Here's how the part is built. I have some questions about the finished solid (model axes, mm). A direction names the side the tool comes from. Round coordinates to 2 decimals unless told otherwise and drop trailing zeros. Loops run counter-clockwise (first coordinate to the right, second up) from the corner with the lowest first, then second, coordinate; pieces in that order, holes last. Notation, with made-up numbers: (-40, 37) -> (-1, 37) arc R12 cw to (-1, 51) -> close; hole circle Ø11 at (-4.75, -33.75). An arc over 180 degrees is marked (long way). Use one line per item in the form item = value. Start each with the question number.
Item 1: If we section it at A-A (z = 8.25): Write out the boundary of the cut face in (x, y), then the cut area to 3 significant figures.
Item 2: If we section it at B-B (x = -3.75): Write out the boundary of the cut face in (y, z), then the cut area to 3 significant figures.
Item 3: If we section it at D-D (x = 11): Write out the boundary of the cut face in (y, z).
Item 4: If I drill on L1, parallel to Z at x = 10.75, y = -0.25; L2, parallel to Z at x = 8, y = -5.75; L3, parallel to X at y = -3.5, z = 4, over which ranges is the centre line in solid material (lowest first)? Write a range as [from, to].
Item 5: For faces 1 (the face through (-7.88, -7.32, 14.38)), 2 (the face through (-1.63, -7.32, 4.87)), 3 (the face through (-7.493, 0.33, 21.869)), 4 (the face through (9.119, 0.33, 20.243)), which set-ups out of +Z, -Z, +X, -X, +Y, -Y let a thin tool reach every point of the face, with its end or its side?
Item 6: I'm going to push flat-ended pins straight in: pin 1 Ø2 at (x, z) = (-1.5, 10) entering from -Y; pin 2 Ø4 at (x, y) = (7, -5.5) entering from +Z; pin 3 Ø1 at (x, z) = (4, 12) entering from +Y; pin 4 Ø1.5 at (x, z) = (2, 22.5) entering from +Y. Where does each tip first touch, or does it pass through?
Item 7: If we section it at C-C (y = 0): Write out the boundary of the cut face in (x, z).
```python
from build123d import *

# Parameters (mm, degrees)
SKETCH1_R                = 7.5
BOSS_EXTRUDE1_DEPTH      = 25.5
BOSS_EXTRUDE2_DEPTH      = 12.75
BOSS_EXTRUDE2_DEPTH_BACK = 12.75
SKETCH2_R                = 7.5


with BuildPart() as part:
    # Sketch1 → Boss-Extrude1 (new body)
    with BuildSketch(Plane.XY):
        Circle(SKETCH1_R)
    extrude(amount=BOSS_EXTRUDE1_DEPTH)

    # Sketch2 → Boss-Extrude2 (add, two sides: drawn at the far end of the back side and taken through both)
    with BuildSketch(Plane(origin=(0, 0, 0), x_dir=(0, 0, -1), z_dir=(1, 0, 0)).offset(-BOSS_EXTRUDE2_DEPTH_BACK)):
        with Locations((-12.75, 0)):
            Circle(SKETCH2_R)
    extrude(amount=BOSS_EXTRUDE2_DEPTH + BOSS_EXTRUDE2_DEPTH_BACK)


solid = part.part
```
Values found:
q1.outline = (-12.75, -6) -> (-4.5, -6) arc R7.5 ccw to (4.5, -6) -> (12.75, -6) -> (12.75, 6) -> (4.5, 6) arc R7.5 ccw to (-4.5, 6) -> (-12.75, 6) -> close
q1.area = 324 mm2
q2.outline = (-6.5, 0) -> (6.5, 0) -> (6.5, 9) arc R7.5 ccw to (6.5, 16.5) -> (6.5, 25.5) -> (-6.5, 25.5) -> (-6.5, 16.5) arc R7.5 ccw to (-6.5, 9) -> close
q2.area = 341 mm2
q3.outline = circle Ø15 at (0, 12.75)
q4.L1 = [5.25, 20.25]
q4.L2 = [7.93, 17.57]
q4.L3 = [-6.63, 6.63]
q5.face_1 = -X
q5.face_2 = -Z
q5.face_3 = +Z
q5.face_4 = +X
q6.pin_1 = -7.48
q6.pin_2 = 25.5
q6.pin_3 = 7.5
q6.pin_4 = 7.4
q7.outline = (-12.75, 5.25) -> (-7.5, 5.25) -> (-7.5, 0) -> (7.5, 0) -> (7.5, 5.25) -> (12.75, 5.25) -> (12.75, 20.25) -> (7.5, 20.25) -> (7.5, 25.5) -> (-7.5, 25.5) -> (-7.5, 20.25) -> (-12.75, 20.25) -> close
